Verification items for the finished model (mm, model axes). A direction names the side the tool comes from. Give positions to 0.01 mm unless a question says otherwise; leave off trailing zeros. Order: outer loops, then holes, each group sorted by start corner. A loop starts at its lowest first (then second) coordinate and runs counter-clockwise, first axis right, second up. Notation, with made-up numbers: (-9, 53) -> (17, 53) arc R14 ccw to (17, 57) -> close; hole circle Ø9 at (89.25, 73). An arc over 180 degrees is marked (long way). Write each question's results on one line, items separated by ' | '. Start each with the question number.
1. Material ranges on L1, parallel to Y at x = -6, z = -1.85; L2, parallel to X at y = -3.5, z = -3.75; L3, parallel to Z at x = 0, y = 2.75, recorded low to high. Write a range as from..to.
2. Cross-section at C-C, the plane x = -6. Enter the section's corners in (y, z).
3. Cross-section at B-B, the plane y = 4. Enter the section's corners in (x, z), then the cut area to 3 significant figures.
4. Cross-section at D-D, the plane y = -7. Enter the section's corners in (x, z), then the cut area to 3 significant figures.
5. Mould release check, pull along X, two halves, no side actions. Record for faces 4 (the face through (8.5, 0, -3)), 5 (the face through (0, 0, -3.2)), 6 (the face through (0, 11.25, -2)): +X half, -X half, draft (parallel to the pull), parting line (faces both ways), or undercut.
6. Cross-section at A-A, the plane z = -6. Enter the section's corners in (x, y).
7. Set-up check for faces 1 (the face through (-3.5, 0, -5)), 2 (the face through (-6, 4, -2.5)), 3 (the face through (-8.5, 0, -3)): record each of +Z, -Z, +X, -X, +Y, -Y from which the full face is reachable in a straight line by a thin tool's end or side.
8. Depth check by flat-ended pin: pin 1 Ø2 at (x, y) = (-0.5, 1.5) entering from -Z; pin 2 Ø0.6 at (x, y) = (-6, 3.5) entering from +Z. Enter the tip coordinate at first touch or a pass-through.
from build123d import *

# Parameters (mm, degrees)
SKETCH1_W           = 17
SKETCH1_H           = 22.5
BOSS_EXTRUDE1_DEPTH = 6.5
SKETCH2_R           = 1
CUT_EXTRUDE1_DEPTH  = 2.5
SKETCH3_W           = 7
SKETCH3_H           = 6.6
CUT_EXTRUDE2_DEPTH  = 25.914855007


with BuildPart() as part:
    # Sketch1 → Boss-Extrude1 (new body)
    with BuildSketch(Plane.XY):
        Rectangle(SKETCH1_W, SKETCH1_H)
    extrude(amount=-BOSS_EXTRUDE1_DEPTH)

    # Sketch2 → Cut-Extrude1 (cut)
    with BuildSketch(Plane.XY):
        with Locations((6, 4)):
            Circle(SKETCH2_R)
        with Locations((6, -4)):
            Circle(SKETCH2_R)
        with Locations((-6, -4)):
            Circle(SKETCH2_R)
        with Locations((-6, 4)):
            Circle(SKETCH2_R)
    extrude(amount=-CUT_EXTRUDE1_DEPTH, mode=Mode.SUBTRACT)

    # Sketch3 → Cut-Extrude2 (cut, through all)
    with BuildSketch(Plane.XZ.offset(11.25)):
        with Locations((0, -6.5)):
            Rectangle(SKETCH3_W, SKETCH3_H)
    extrude(amount=-CUT_EXTRUDE2_DEPTH, mode=Mode.SUBTRACT)


solid = part.part
Results below:
1) L1: y = -11.25..-5, -3..3, 5..11.25 | L2: x = -8.5..-3.5, 3.5..8.5 | L3: z = -3.2..0
2) outline: (-11.25, -6.5) -> (11.25, -6.5) -> (11.25, 0) -> (5, 0) -> (5, -2.5) -> (3, -2.5) -> (3, 0) -> (-3, 0) -> (-3, -2.5) -> (-5, -2.5) -> (-5, 0) -> (-11.25, 0) -> close
3) outline: (-8.5, -6.5) -> (-3.5, -6.5) -> (-3.5, -3.2) -> (3.5, -3.2) -> (3.5, -6.5) -> (8.5, -6.5) -> (8.5, 0) -> (7, 0) -> (7, -2.5) -> (5, -2.5) -> (5, 0) -> (-5, 0) -> (-5, -2.5) -> (-7, -2.5) -> (-7, 0) -> (-8.5, 0) -> close | area: 77.4 mm²
4) outline: (-8.5, -6.5) -> (-3.5, -6.5) -> (-3.5, -3.2) -> (3.5, -3.2) -> (3.5, -6.5) -> (8.5, -6.5) -> (8.5, 0) -> (-8.5, 0) -> close | area: 87.4 mm²
5) face 4: +X half | face 5: undercut | face 6: draft
6) outline: (-8.5, -11.25) -> (-3.5, -11.25) -> (-3.5, 11.25) -> (-8.5, 11.25) -> close; (3.5, -11.25) -> (8.5, -11.25) -> (8.5, 11.25) -> (3.5, 11.25) -> close
7) face 1: -Z, +Y, -Y | face 2: +Z | face 3: +Z, -Z, -X, +Y, -Y
8) pin 1: stops at z = -3.2 | pin 2: stops at z = -2.5
